Model file for the job. Use its own axes, mm. Round coordinates to 2 decimals unless told otherwise and drop trailing zeros. Order: outer loops, then holes, each group sorted by start corner. A loop starts at its lowest first (then second) coordinate and runs counter-clockwise, first axis right, second up. Notation, with made-up numbers: (-9, -8) - (23, -8) arc R23 cw to (23, 16) - close; hole circle Ø6 at (88.5, -22.75). An arc over 180 degrees is marked (long way). Write item = value, one per line.
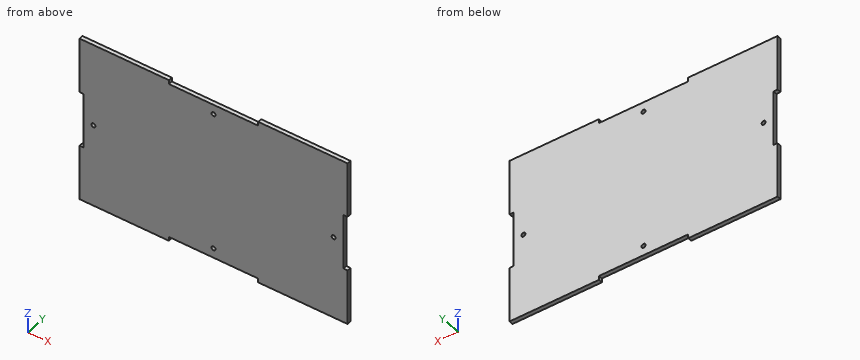
```python
from build123d import *

# Parameters (mm, degrees)
F0_R     = 1.5
F1_DEPTH = 3


with BuildPart() as f1:
    # F0 (on Front) → F1 (new body)
    with BuildSketch(Plane.XZ):
        Polygon((-100, -20.833333), (-100, -62.5), (-33.333333, -62.5), (-33.333333, -59.5), (33.333333, -59.5), (33.333333, -62.5), (100, -62.5), (100, -20.833333), (97, -20.833333), (97, 20.833333), (100, 20.833333), (100, 62.5), (33.333333, 62.5), (33.333333, 59.5), (-33.333333, 59.5), (-33.333333, 62.5), (-100, 62.5), (-100, 20.833333), (-97, 20.833333), (-97, -20.833333), align=None)
        with Locations((0, -52.2)):
            Circle(F0_R, mode=Mode.SUBTRACT)
        with Locations((-89.7, 0)):
            Circle(F0_R, mode=Mode.SUBTRACT)
        with Locations((89.7, 0)):
            Circle(F0_R, mode=Mode.SUBTRACT)
        with Locations((0, 52.2)):
            Circle(F0_R, mode=Mode.SUBTRACT)
    extrude(amount=F1_DEPTH)


with BuildPart() as f2_1:
    # F2: copy of F1
    add(f1.part.moved(Location((0, 60, 0))))


solid = f1.part
```
1) Cut at B-B (z = -11). Write the cut outline in (x, y).
Conclusion:
outline = (-97, -3) - (97, -3) - (97, 0) - (-97, 0) - close
2) Cut at A-A (y = -0.6). Write the cut outline in (x, z).
Conclusion:
outline = (-100, -62.5) - (-33.33, -62.5) - (-33.33, -59.5) - (33.33, -59.5) - (33.33, -62.5) - (100, -62.5) - (100, -20.83) - (97, -20.83) - (97, 20.83) - (100, 20.83) - (100, 62.5) - (33.33, 62.5) - (33.33, 59.5) - (-33.33, 59.5) - (-33.33, 62.5) - (-100, 62.5) - (-100, 20.83) - (-97, 20.83) - (-97, -20.83) - (-100, -20.83) - close; hole circle Ø3 at (-89.7, 0); hole circle Ø3 at (0, -52.2); hole circle Ø3 at (0, 52.2); hole circle Ø3 at (89.7, 0)
3) Wall check: line 1 along Z through (x, y) = (0, -0.9); line 2 along Z through (x, y) = (89.7, -0.85); line 3 along X through (y, z) = (-0.5, -10.5). Give the ranges that are in metal, low to high.
Conclusion:
line_1 = -59.5 to -53.7, -50.7 to 50.7, 53.7 to 59.5
line_2 = -62.5 to -1.5, 1.5 to 62.5
line_3 = -97 to 97
4) Flat gauge pins, fed straight in: pin 1 Ø5 at (x, z) = (89.7, 0) entering from -Y; pin 2 Ø1.5 at (y, z) = (-2, 4.5) entering from -X; pin 3 Ø1.5 at (x, y) = (-7.5, -1) entering from -Z. Where does each tip first touch, or does it go through?
Conclusion:
pin_1 = -3
pin_2 = -97
pin_3 = -59.5
5) Cut at C-C (x = 10). Write the cut outline in (y, z).
Conclusion:
outline = (-3, -59.5) - (0, -59.5) - (0, 59.5) - (-3, 59.5) - close
